Answer from the drawing. Dimensions are ordinates in mm from the lowest x, y and z of the part. A direction names the side the tool comes from. Give positions to 0.01 mm unless a question says otherwise; leave off trailing zeros. Order: outer loops, then holes, each group sorted by start corner. A loop starts at its lowest first (then second) coordinate and runs counter-clockwise, first axis right, second up.
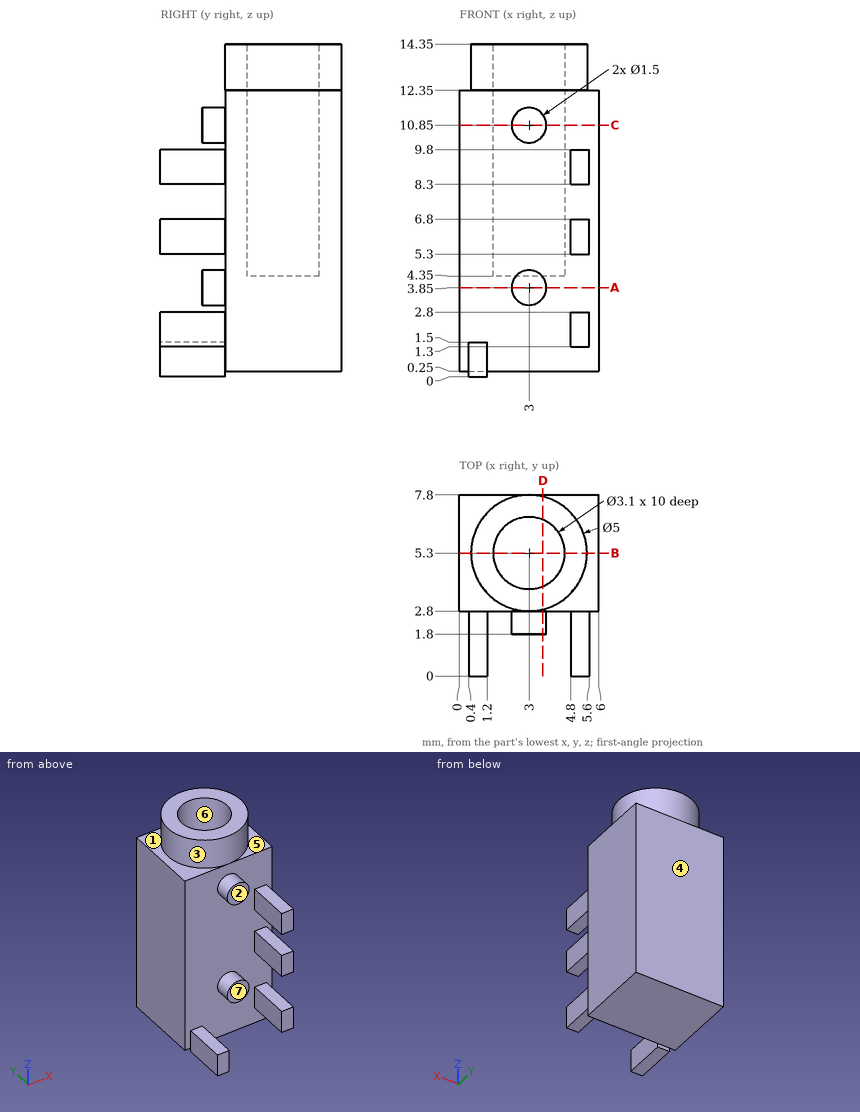
1. The part is cut by section B-B (y = 5.3). Write down the section's boundary in (x, z).
Findings below:
outline: (0, 0.25) - (6, 0.25) - (6, 12.35) - (5.5, 12.35) - (5.5, 14.35) - (4.55, 14.35) - (4.55, 4.35) - (1.45, 4.35) - (1.45, 14.35) - (0.5, 14.35) - (0.5, 12.35) - (0, 12.35) - close
2. The part is cut by section A-A (z = 3.85). Write down the section's boundary in (x, y), then the cut area to 3 significant figures.
Findings below:
outline: (0, 2.8) - (2.25, 2.8) - (2.25, 1.8) - (3.75, 1.8) - (3.75, 2.8) - (6, 2.8) - (6, 7.8) - (0, 7.8) - close
area: 31.5 mm2
3. Which of the six approach directions +Z, -Z, +X, -X, +Y, -Y give full straight-line access (tool end or side, diameter ignored) to the marked faces 1, 2 and 3?
Findings below:
face 1: +Z, -X
face 2: +Z, -Z, +X, -X, -Y
face 3: +Z
4. The part is cut by section C-C (z = 10.85). Write down the section's boundary in (x, y), then the cut area to 3 significant figures.
Findings below:
outline: (0, 2.8) - (2.25, 2.8) - (2.25, 1.8) - (3.75, 1.8) - (3.75, 2.8) - (6, 2.8) - (6, 7.8) - (0, 7.8) - close; hole circle Ø3.1 at (3, 5.3)
area: 24.0 mm2
5. Given P1, Ø0.8, axis at y = 1, z = 6, coming from the +X side; P2, Ø0.8, axis at y = 2, z = 9.5, coming from the -X side; P3, Ø2.5, axis at x = 2.5, y = 5.5, coming from the +Z side; P4, Ø1.2, axis at y = 2, z = 0.5, coming from the +X side, each flat-ended and moving along its own axis, determine where each tip first touches the part or whether it passes through.
Findings below:
P1: stops at x = 5.6
P2: stops at x = 4.8
P3: stops at z = 14.35
P4: stops at x = 1.2
6. Straight lines are drawn through the part: probe 1 along Y at (x, z) = (3, 9.5); probe 2 along Y at (x, z) = (1.3, 5.25); probe 3 along Z at (x, y) = (3.2, 3). For each, find the intervals that lie inside material, in ascending order.
Findings below:
probe 1: y = 2.8 to 3.75, 6.85 to 7.8
probe 2: y = 2.8 to 7.8
probe 3: z = 0.25 to 14.35
7. The part is cut by section D-D (x = 3.6). Write down the section's boundary in (y, z), then the cut area to 3 significant figures.
Findings below:
outline: (1.8, 3.4) - (2.8, 3.4) - (2.8, 0.25) - (7.8, 0.25) - (7.8, 12.35) - (7.73, 12.35) - (7.73, 14.35) - (6.73, 14.35) - (6.73, 4.35) - (3.87, 4.35) - (3.87, 14.35) - (2.87, 14.35) - (2.87, 12.35) - (2.8, 12.35) - (2.8, 11.3) - (1.8, 11.3) - (1.8, 10.4) - (2.8, 10.4) - (2.8, 4.3) - (1.8, 4.3) - close
area: 43.4 mm2
8. The mould has two halves that part along Y. Classify the marked faces 4, 5, 6 and 7: pulls with the +Y half, pulls with the -Y half, needs draft (parallel to the pull), parting line crosses it, or undercut.
Findings below:
face 4: pulls with the +Y half
face 5: needs draft
face 6: undercut
face 7: pulls with the -Y half
